Can you work these out from the model? Positions are in its coordinate system, mm. Face numbers are marked on the shaded views. Coordinates: 2 decimals unless noted, no trailing zeros. Order: outer loops, then holes, each group sorted by start corner. A loop starts at its lowest first (then second) coordinate and runs counter-clockwise, first axis right, second up. Notation, with made-up numbers: (24, -12) -> (28, -12) arc R28 ccw to (28, 11) -> close; hole circle Ø10 at (32, -22). An arc over 180 degrees is marked (long way). Answer as a JSON object with one key per item and string values. Group by question number.
(1) For pin 1 (3 mm diameter, centred on x = 21.5, z = 23, fed in from +Y); pin 2 (6 mm diameter, centred on x = -18, z = 10.5, fed in from +Y); pin 3 (1 mm diameter, centred on y = -1, z = 8, fed in from -X); pin 4 (1.5 mm diameter, centred on x = -21.5, y = -10, fed in from +Z), each with a flat end and sliding along its axis, tell me the tip position at first contact or that it passes through.
(2) If we mould it in two halves opening along Y, with no side actions, what happens to the marked faces 1 and 2? For each: pulls with the +Y half, pulls with the -Y half, needs draft (parallel to the pull), parting line crosses it, or undercut.
(3) I want a section at A-A, the plane y = 0. List the corners of the cut face in (x, z) for me (1 decimal), plus the area to 3 significant figures.
(4) I want a section at C-C, the plane z = 23.5. List the corners of the cut face in (x, y) for me.
(5) I want a section at D-D, the plane z = 2. List the corners of the cut face in (x, y) for me.
(6) I need wall thicknesses on line 1 (Y direction, x = 0, z = 10); line 2 (X direction, y = -15, z = 24); line 3 (X direction, y = -2, z = 7.75). Which ranges of each line are inside material? Lowest first, please.
from build123d import *

# Parameters (mm, degrees)
F0_R     = 29.8077198066
F1_DEPTH = 25.4
F2_R     = 26.3502536292
F3_DEPTH = 25.4
F4_W     = 2.8885006905
F4_H     = 0.9121578187


# Not quite as in the source:
# - a fillet or chamfer that OpenCascade refuses, or shapes differently, is made with other operations: its cross-section is extruded or revolved along the edge and cut away or added


with BuildPart() as f1:
    # F0 (on Top) → F1 (new body)
    with BuildSketch(Plane.XY):
        Circle(F0_R)
    extrude(amount=F1_DEPTH)

    # F2 (on face) → F3 (cut)
    with BuildSketch(Plane.XY.offset(25.4)):
        Circle(F2_R)
    extrude(amount=-F3_DEPTH, mode=Mode.SUBTRACT)

    # F4 (on Right) → F6 (revolve, cut)
    with BuildSketch(Plane.YZ):
        with Locations((-30.5377691984, 14.828927815)):
            Rectangle(F4_W, F4_H)
    revolve(axis=Axis((0, 0, 31.8907126784), (0, 0, 1)), mode=Mode.SUBTRACT)

    # F7: fillet of radius 5.08 on 6 edges, made by hand

    # F7_s1 → F7_t2 (revolve, cut)
    with BuildSketch(Plane.XZ):
        with BuildLine():
            ThreePointArc((29.0935188532, 15.2850067243), (29.6259163705, 16.5354769537), (29.8077198066, 17.8823512692))
            Line((29.8077198066, 17.8823512692), (29.9093198066, 17.8823512692))
            Line((29.9093198066, 17.8823512692), (29.9093198066, 15.2850067243))
            Line((29.9093198066, 15.2850067243), (29.8077198066, 15.1834067243))
            ThreePointArc((29.8077198066, 15.1834067243), (29.4506193299, 15.1834067243), (29.1808348341, 15.2330598334))
            Line((29.1808348341, 15.2330598334), (29.0935188532, 15.2850067243))
        make_face()
    revolve(axis=Axis((0, 0, 15.2850067243), (0, 0, -1)), mode=Mode.SUBTRACT)

    # F7_s3 → F7_t4 (revolve, cut)
    with BuildSketch(Plane.XZ):
        with BuildLine():
            ThreePointArc((26.3502536292, 25.4), (28.8537876574, 23.5495222224), (29.8077198066, 20.5860843387))
            Line((29.8077198066, 20.5860843387), (29.9093198066, 20.5860843387))
            Line((29.9093198066, 20.5860843387), (29.9093198066, 25.4))
            Line((29.9093198066, 25.4), (29.8077198066, 25.5016))
            ThreePointArc((29.8077198066, 25.5016), (28.0789867179, 25.5016), (26.3827043057, 25.4962783132))
            Line((26.3827043057, 25.4962783132), (26.3502536292, 25.4))
        make_face()
    revolve(axis=Axis((0, 0, 25.4), (0, 0, 1)), mode=Mode.SUBTRACT)

    # F7_s5 → F7_t6 (revolve, cut)
    with BuildSketch(Plane.XZ):
        with BuildLine():
            ThreePointArc((29.8077198066, 4.8139156613), (28.8537876574, 1.8504777776), (26.3502536292, 0))
            Line((26.3502536292, 0), (26.3827043057, -0.0962783132))
            ThreePointArc((26.3827043057, -0.0962783132), (28.0789867179, -0.1016), (29.8077198066, -0.1016))
            Line((29.8077198066, -0.1016), (29.9093198066, 0))
            Line((29.9093198066, 0), (29.9093198066, 4.8139156613))
            Line((29.9093198066, 4.8139156613), (29.8077198066, 4.8139156613))
        make_face()
    revolve(axis=Axis((0, 0, 0), (0, 0, 1)), mode=Mode.SUBTRACT)

    # F7_s7 → F7_t8 (revolve, cut)
    with BuildSketch(Plane.XZ):
        with BuildLine():
            ThreePointArc((29.8077198066, 11.7755043607), (29.6259163705, 13.1223786762), (29.0935188532, 14.3728489056))
            Line((29.0935188532, 14.3728489056), (29.1808348341, 14.4247957965))
            ThreePointArc((29.1808348341, 14.4247957965), (29.4506193299, 14.4744489056), (29.8077198066, 14.4744489056))
            Line((29.8077198066, 14.4744489056), (29.9093198066, 14.3728489056))
            Line((29.9093198066, 14.3728489056), (29.9093198066, 11.7755043607))
            Line((29.9093198066, 11.7755043607), (29.8077198066, 11.7755043607))
        make_face()
    revolve(axis=Axis((0, 0, 14.3728489056), (0, 0, -1)), mode=Mode.SUBTRACT)


solid = f1.part
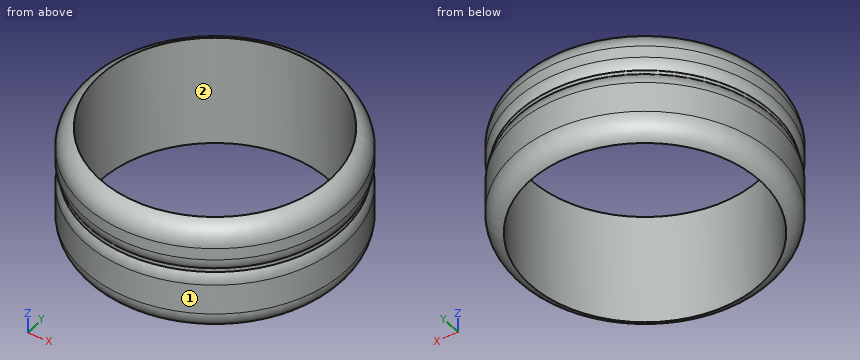
Computed values:
{
 "1": {"pin 1": "stops at y = 21.54", "pin 2": "stops at y = 25.76", "pin 3": "stops at x = -29.8", "pin 4": "passes through"},
 "2": {"face 1": "parting line crosses it", "face 2": "undercut"},
 "3": {"outline": "(-29.8, 4.8) arc R5.1 ccw to (-26.4, 0) -> (-26.4, 25.4) arc R5.1 ccw to (-29.8, 20.6) -> (-29.8, 17.9) arc R5.1 ccw to (-29.1, 15.3) -> (-29.1, 14.4) arc R5.1 ccw to (-29.8, 11.8) -> close; (26.4, 0) arc R5.1 ccw to (29.8, 4.8) -> (29.8, 11.8) arc R5.1 ccw to (29.1, 14.4) -> (29.1, 15.3) arc R5.1 ccw to (29.8, 17.9) -> (29.8, 20.6) arc R5.1 ccw to (26.4, 25.4) -> close", "area": "154 mm2"},
 "4": {"outline": "circle Ø57.78 at (0, 0); hole circle Ø52.7 at (0, 0)"},
 "5": {"outline": "circle Ø57.91 at (0, 0); hole circle Ø52.7 at (0, 0)"},
 "6": {"line 1": "y = -29.81 to -26.35, 26.35 to 29.81", "line 2": "x = -24.22 to -21.66, 21.66 to 24.22", "line 3": "x = -29.74 to -26.27, 26.27 to 29.74"}
}
